The drawing under review shows one solid part. Ordinate dimensions are in mm from its lowest x, y, z. Coordinates: 2 decimals unless noted, no trailing zeros. Loops run counter-clockwise (first coordinate to the right, second up) from the corner with the lowest first, then second, coordinate; pieces in that order, holes last.
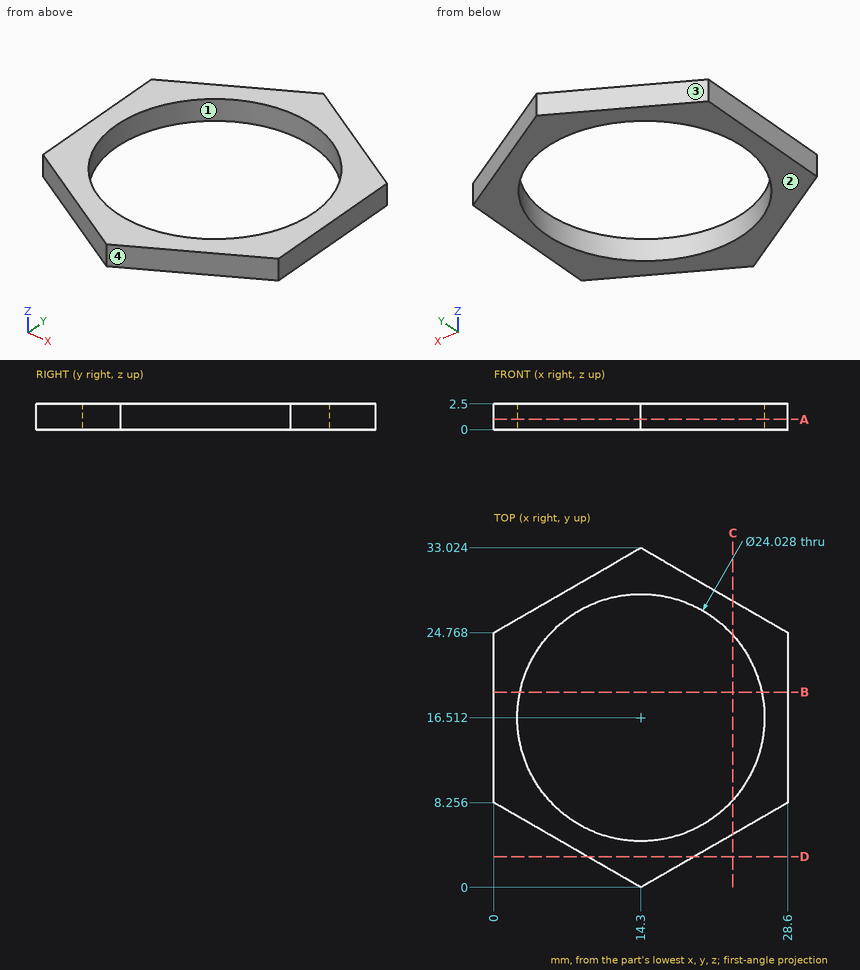
Q1. Take a section at D-D, the plane y = 3. Write out the cut boundary in (x, z).
Q2. The part is to be moulded in two halves that separate along X. For the marked faces 1, 2, 3 and 4, say which applies: pulls with the +X half, pulls with the -X half, needs draft (parallel to the pull), parting line crosses it, or undercut.
Q3. Take a section at A-A, the plane z = 1. Write out the cut boundary in (x, y) (1 decimal).
Q4. Take a section at C-C, the plane x = 23.25. Write out the cut boundary in (y, z).
Q5. Take a section at B-B, the plane y = 19. Write out the cut boundary in (x, z), then the cut area to 3 significant figures.
Q6. Clearance check with flat-ended pins moving along their axes: pin 1 Ø1 at (y, z) = (27, 1) entering from -X; pin 2 Ø1.5 at (x, z) = (7.5, 2) entering from +Y. State where each tip first meets the part, or that it passes through.
Q7. For line 1 (X direction, y = 17, z = 1.85) (1 decimal); line 2 (X direction, y = 14, z = 1.7); line 3 (Y direction, x = 10.5, z = 2.2) (1 decimal), list the stretches that pass through material, from the lowest coordinate up.
Entries:
1. outline: (9.1, 0) - (19.5, 0) - (19.5, 2.5) - (9.1, 2.5) - close
2. face 1: undercut
2. face 2: needs draft
2. face 3: pulls with the -X half
2. face 4: pulls with the +X half
3. outline: (0, 8.3) - (14.3, 0) - (28.6, 8.3) - (28.6, 24.8) - (14.3, 33) - (0, 24.8) - close; hole circle Ø24 at (14.3, 16.5)
4. outline: (5.17, 0) - (8.5, 0) - (8.5, 2.5) - (5.17, 2.5) - close; (24.53, 0) - (27.86, 0) - (27.86, 2.5) - (24.53, 2.5) - close
5. outline: (0, 0) - (2.55, 0) - (2.55, 2.5) - (0, 2.5) - close; (26.05, 0) - (28.6, 0) - (28.6, 2.5) - (26.05, 2.5) - close
5. area: 12.7 mm2
6. pin 1: stops at x = 3
6. pin 2: stops at y = 29.53
7. line 1: x = 0 to 2.3, 26.3 to 28.6
7. line 2: x = 0 to 2.55, 26.05 to 28.6
7. line 3: y = 2.2 to 5.1, 27.9 to 30.8
